from build123d import *

# Parameters (mm, degrees)
BOSS_EXTRUDE1_DEPTH  = 5
M3_CLEARANCE_HOLE2_D = 3.4


with BuildPart() as part:
    # Sketch1 → Boss-Extrude1 (new body)
    with BuildSketch(Plane.XY):
        Polygon((8.235294118, 15.882352941), (8.235294118, 18.882352941), (-6.764705882, 18.882352941), (-6.764705882, 14.294117647), (-6.764705882, -25.352941176), (-6.764705882, -31.117647059), (-0.882352941, -31.117647059), (8.235294118, -31.117647059), (8.235294118, -28.117647059), (-0.764705882, -28.117647059), (-0.764705882, 15.882352941), align=None)
    extrude(amount=BOSS_EXTRUDE1_DEPTH)

    # M3 Clearance Hole2 (through all)
    with Locations(Plane.XY.offset(5)):
        with Locations((-3.858851748, 13.882352941), (-3.858851748, -26.117647059)):
            Hole(M3_CLEARANCE_HOLE2_D / 2)


solid = part.part
Read the model definition and answer for the solid it produces. Units are mm, in the model's axes. A direction names the side the tool comes from. Coordinates: 2 decimals unless noted, no trailing zeros. Write each loop counter-clockwise with the first axis right and the second up, starting at its lowest first coordinate (ties: lowest second). Pieces come first, ordered by that corner, then holes. Notation, with made-up numbers: M -27,8.25 L -17,8.25 A34 ccw -17,43.25 Z; hole C -23,2.25 d2. An arc over 180 degrees is marked long. Use a Markdown table: item, result.
Q1. Which of the six approach directions +Z, -Z, +X, -X, +Y, -Y give full straight-line access (tool end or side, diameter ignored) to faces 5 (the face through (8.235, 17, 2)), 6 (the face through (-0.765, -6, 2))?
Answer block:
| item | result |
|---|---|
| face 5 | +Z, -Z, +X, +Y, -Y |
| face 6 | +Z, -Z, +X |
Q2. Each of these flat-tipped pins is pushed along its axis until it touches: pin 1 Ø2 at (x, y) = (-1, 12.5) entering from -Z; pin 2 Ø2.5 at (x, y) = (-3.86, 13.88) entering from -Z. Where does it stop, or does it pass through?
Answer block:
| item | result |
|---|---|
| pin 1 | stops at z = 0 |
| pin 2 | passes through |
Q3. The part is cut by section C-C, the plane x = -3.75. Write down the section's boundary in (y, z).
Answer block:
| item | result |
|---|---|
| outline | M -31.12,0 L -27.81,0 L -27.81,5 L -31.12,5 Z; M -24.42,0 L 12.19,0 L 12.19,5 L -24.42,5 Z; M 15.58,0 L 18.88,0 L 18.88,5 L 15.58,5 Z |
Q4. Straight lines are drawn through the part: L1, parallel to Y at x = 2, z = 3.3; L2, parallel to X at y = -5, z = 1.9; L3, parallel to Y at x = -3.25, z = 3.65. For each, find the intervals that lie inside material, in ascending order. Write a range as [from, to].
Answer block:
| item | result |
|---|---|
| L1 | y = [-31.12, -28.12], [15.88, 18.88] |
| L2 | x = [-6.76, -0.76] |
| L3 | y = [-31.12, -27.7], [-24.53, 12.3], [15.47, 18.88] |
Q5. The part is cut by section B-B, the plane z = 1.8. Write down the section's boundary in (x, y).
Answer block:
| item | result |
|---|---|
| outline | M -6.76,-31.12 L 8.24,-31.12 L 8.24,-28.12 L -0.76,-28.12 L -0.76,15.88 L 8.24,15.88 L 8.24,18.88 L -6.76,18.88 Z; hole C -3.86,-26.12 d3.4; hole C -3.86,13.88 d3.4 |
Q6. Determine the mould class of faces 1 (the face through (-3.49, 12.223, 2.465)), 2 (the face through (-4.643, -27.626, 2.465)), 3 (the face through (4, -28.118, 2)), 4 (the face through (8.235, -30, 2)) for opening direction X: released by +X, released by -X, zero draft, split by the parting line, or undercut.
Answer block:
| item | result |
|---|---|
| face 1 | undercut |
| face 2 | undercut |
| face 3 | zero draft |
| face 4 | released by +X |
Q7. The part is cut by section A-A, the plane x = 3.75. Write down the section's boundary in (y, z), then the cut area to 3 significant figures.
Answer block:
| item | result |
|---|---|
| outline | M -31.12,0 L -28.12,0 L -28.12,5 L -31.12,5 Z; M 15.88,0 L 18.88,0 L 18.88,5 L 15.88,5 Z |
| area | 30.0 mm2 |
Q8. The part is cut by section D-D, the plane y = -5.5. Write down the section's boundary in (x, z), then the cut area to 3 significant figures.
Answer block:
| item | result |
|---|---|
| outline | M -6.76,0 L -0.76,0 L -0.76,5 L -6.76,5 Z |
| area | 30.0 mm2 |
